```python
from build123d import *

# Parameters (mm, degrees)
F0_W     = 50
F0_H     = 66
F1_DEPTH = 50
F2_W     = 24
F2_H     = 15
F3_DEPTH = 66
F4_R     = 6
F5_DEPTH = 66
F6_W     = 12
F6_H     = 16
F7_DEPTH = 35
F8_W     = 2
F8_H     = 16
F9_DEPTH = 35


with BuildPart() as f1:
    # F0 (on Top) → F1 (new body)
    with BuildSketch(Plane.XY):
        with Locations((25, 33)):
            Rectangle(F0_W, F0_H)
    extrude(amount=F1_DEPTH)

    # F2 (on face) → F3 (cut)
    with BuildSketch(Plane.XZ):
        with Locations((25, 42.5)):
            Rectangle(F2_W, F2_H)
    extrude(amount=-F3_DEPTH, mode=Mode.SUBTRACT)

    # F4 (on face) → F5 (cut)
    with BuildSketch(Plane.XZ):
        with Locations((25, 17)):
            Circle(F4_R)
    extrude(amount=-F5_DEPTH, mode=Mode.SUBTRACT)

    # F6 (on face) → F7 (cut)
    with BuildSketch(Plane.XY.offset(35)):
        with Locations((25, 48)):
            Rectangle(F6_W, F6_H)
        with Locations((25, 18)):
            Rectangle(F6_W, F6_H)
    extrude(amount=-F7_DEPTH, mode=Mode.SUBTRACT)

    # F8 (on face) → F9 (cut)
    with BuildSketch(Plane.XY.offset(35)):
        with Locations((18, 48)):
            Rectangle(F8_W, F8_H)
        with Locations((32, 48)):
            Rectangle(F8_W, F8_H)
        with Locations((18, 18)):
            Rectangle(F8_W, F8_H)
        with Locations((32, 18)):
            Rectangle(F8_W, F8_H)
    extrude(amount=-F9_DEPTH, mode=Mode.SUBTRACT)


solid = f1.part
```
CAD build for the part. Positions are in the model's coordinates, mm. A direction names the side the tool comes from. Round coordinates to 2 decimals unless told otherwise and drop trailing zeros. Loops run counter-clockwise (first coordinate to the right, second up) from the corner with the lowest first, then second, coordinate; pieces in that order, holes last. Notation, with made-up numbers: M 11.5,-17.5 L 65.5,-17.5 A12 cw 65.5,-1.5 Z; hole C 11,21.5 d5. An arc over 180 degrees is marked long. Use a Markdown table: item, result. Add a question column.
(1) Cut at C-C (y = 24.5). Give the cut face in (x, z).
(2) Cut at D-D (z = 17). Give the cut face in (x, y), and give its area (3 significant figures).
(3) Flat gauge pin, fed straight in: pin 1 (7 mm diameter, centred on x = 27, y = 32, fed in from +Z). Where does the tip first touch, or does it go through?
(4) Cut at A-A (z = 26.5). Give the cut face in (x, y).
(5) Drill centre lines: line 1 (X direction, y = 35.5, z = 17); line 2 (Y direction, x = 19.5, z = 31.5); line 3 (X direction, y = 11, z = 28.5). Where is each one in solid material? Low to high.
(6) Which spindle directions (+Z, -Z, +X, -X, +Y, -Y) get a long thin tool onto all of the face, cutting with end or side? Do faces 1 (the face through (43, 33, 50)), 2 (the face through (19.6, 40, 13.9)), 3 (the face through (25, 33, 35)). Say none if no direction does.
(7) Pull direction Y, two halves, no side cores. Call faces 4 (the face through (25, 66, 25)), 5 (the face through (33, 18, 18)), 6 (the face through (19, 33, 17)): +Y half, -Y half, draft (parallel to the pull), parting line (faces both ways), or undercut.
(8) Cut at B-B (x = 25). Give the cut face in (y, z).
Geometry says:
| question | item | result |
|---|---|---|
| 1 | outline | M 0,0 L 17,0 L 17,35 L 13,35 L 13,50 L 0,50 Z; M 33,0 L 50,0 L 50,50 L 37,50 L 37,35 L 33,35 Z |
| 2 | outline | M 0,0 L 19,0 L 19,10 L 17,10 L 17,26 L 19,26 L 19,40 L 17,40 L 17,56 L 19,56 L 19,66 L 0,66 Z; M 31,0 L 50,0 L 50,66 L 31,66 L 31,56 L 33,56 L 33,40 L 31,40 L 31,26 L 33,26 L 33,10 L 31,10 Z |
| 2 | area | 2,380 mm² |
| 3 | pin 1 | stops at z = 35 |
| 4 | outline | M 0,0 L 50,0 L 50,66 L 0,66 Z; hole M 17,10 L 33,10 L 33,26 L 17,26 Z; hole M 17,40 L 33,40 L 33,56 L 17,56 Z |
| 5 | line 1 | x = 0 to 19, 31 to 50 |
| 5 | line 2 | y = 0 to 10, 26 to 40, 56 to 66 |
| 5 | line 3 | x = 0 to 17, 33 to 50 |
| 6 | face 1 | +Z, +X, -X, +Y, -Y |
| 6 | face 2 | +Z, -Z |
| 6 | face 3 | +Z, +Y, -Y |
| 7 | face 4 | +Y half |
| 7 | face 5 | undercut |
| 7 | face 6 | draft |
| 8 | outline | M 0,0 L 10,0 L 10,11 L 0,11 Z; M 0,23 L 10,23 L 10,35 L 0,35 Z; M 26,0 L 40,0 L 40,11 L 26,11 Z; M 26,23 L 40,23 L 40,35 L 26,35 Z; M 56,0 L 66,0 L 66,11 L 56,11 Z; M 56,23 L 66,23 L 66,35 L 56,35 Z |
